Geometry: see drawing. Coordinates: mm, zero at the bounding-box minimum. Round coordinates to 2 decimals unless told otherwise and drop trailing zeros. Loops run counter-clockwise (first coordinate to the right, second up) from the corner with the lowest first, then second, coordinate; pieces in that order, holes last.
(1) Section A-A, the plane x = 77.3. Return the cut outline in (y, z).
(2) Section D-D, the plane z = 1.95. Return the cut outline in (x, y).
(3) Material intervals for probe 1 along X at (y, z) = (42.7, 1.7); probe 2 along Y at (x, z) = (77.3, 2); probe 3 along Y at (x, z) = (12.7, 1.1), sorted ascending.
(4) Section C-C, the plane y = 42.7. Return the cut outline in (x, z).
(5) Section B-B, the plane y = 87.3. Return the cut outline in (x, z).
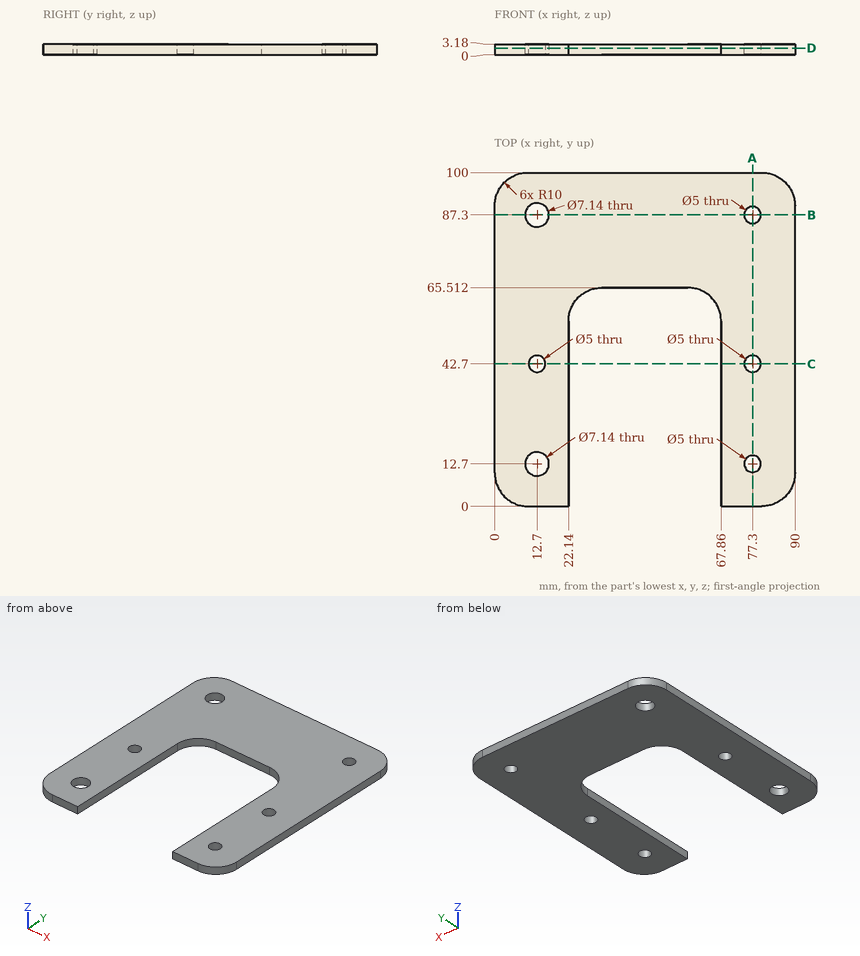
Output values:
1. outline: (0, 0) - (10.2, 0) - (10.2, 3.18) - (0, 3.18) - close; (15.2, 0) - (40.2, 0) - (40.2, 3.18) - (15.2, 3.18) - close; (45.2, 0) - (84.8, 0) - (84.8, 3.18) - (45.2, 3.18) - close; (89.8, 0) - (100, 0) - (100, 3.18) - (89.8, 3.18) - close
2. outline: (0, 10) arc R10 ccw to (10, 0) - (22.14, 0) - (22.14, 55.51) arc R10 cw to (32.14, 65.51) - (57.86, 65.51) arc R10 cw to (67.86, 55.51) - (67.86, 0) - (80, 0) arc R10 ccw to (90, 10) - (90, 90) arc R10 ccw to (80, 100) - (10, 100) arc R10 ccw to (0, 90) - close; hole circle Ø7.14 at (12.7, 12.7); hole circle Ø7.14 at (12.7, 87.3); hole circle Ø5 at (12.7, 42.7); hole circle Ø5 at (77.3, 12.7); hole circle Ø5 at (77.3, 42.7); hole circle Ø5 at (77.3, 87.3)
3. probe 1: x = 0 to 10.2, 15.2 to 22.14, 67.86 to 74.8, 79.8 to 90
3. probe 2: y = 0 to 10.2, 15.2 to 40.2, 45.2 to 84.8, 89.8 to 100
3. probe 3: y = 0 to 9.13, 16.27 to 40.2, 45.2 to 83.73, 90.87 to 100
4. outline: (0, 0) - (10.2, 0) - (10.2, 3.18) - (0, 3.18) - close; (15.2, 0) - (22.14, 0) - (22.14, 3.18) - (15.2, 3.18) - close; (67.86, 0) - (74.8, 0) - (74.8, 3.18) - (67.86, 3.18) - close; (79.8, 0) - (90, 0) - (90, 3.18) - (79.8, 3.18) - close
5. outline: (0, 0) - (9.13, 0) - (9.13, 3.18) - (0, 3.18) - close; (16.27, 0) - (74.8, 0) - (74.8, 3.18) - (16.27, 3.18) - close; (79.8, 0) - (90, 0) - (90, 3.18) - (79.8, 3.18) - close
